Geometry: see drawing. Coordinates: mm, zero at the bounding-box minimum. Round coordinates to 2 decimals unless told otherwise and drop trailing zeros. Order: outer loops, then holes, each group sorted by start corner. A loop starts at its lowest first (then second) coordinate and runs counter-clockwise, first axis right, second up. Notation, with made-up numbers: (18.25, -8.5) -> (72.25, -8.5) arc R13 cw to (72.25, 16.5) -> close; hole circle Ø6 at (40.25, 57.5). An arc over 180 degrees is marked (long way). Answer as CSV lines item,"result". Start each with the question number.
(1) Section query B-B (y = 10.16). Output: boundary loops of the cut face in (x, z) (3 decimals).
(2) Section query A-A (x = 12.7). Output: boundary loops of the cut face in (y, z) (3 decimals).
(3) Section query C-C (z = 2.45). Output: boundary loops of the cut face in (x, y), plus the area to 3 significant figures.
(4) Line query: line 1 along Y through (x, z) = (38.1, 0.9); line 2 along X through (y, z) = (10.16, 0.7); line 3 along Y through (x, z) = (39.5, 2.4). Output: solid intervals per line, ascending. Write a range as from..to.
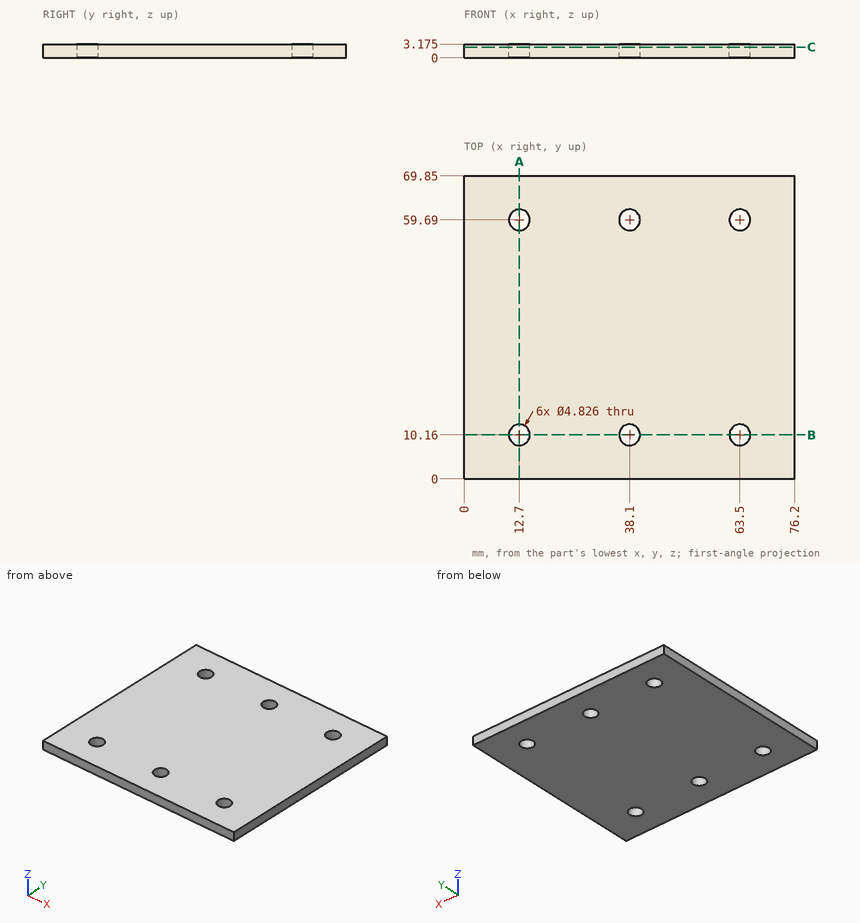
Answer block:
1,outline,"(0, 0) -> (10.287, 0) -> (10.287, 3.175) -> (0, 3.175) -> close; (15.113, 0) -> (35.687, 0) -> (35.687, 3.175) -> (15.113, 3.175) -> close; (40.513, 0) -> (61.087, 0) -> (61.087, 3.175) -> (40.513, 3.175) -> close; (65.913, 0) -> (76.2, 0) -> (76.2, 3.175) -> (65.913, 3.175) -> close"
2,outline,"(0, 0) -> (7.747, 0) -> (7.747, 3.175) -> (0, 3.175) -> close; (12.573, 0) -> (57.277, 0) -> (57.277, 3.175) -> (12.573, 3.175) -> close; (62.103, 0) -> (69.85, 0) -> (69.85, 3.175) -> (62.103, 3.175) -> close"
3,outline,"(0, 0) -> (76.2, 0) -> (76.2, 69.85) -> (0, 69.85) -> close; hole circle Ø4.83 at (12.7, 10.16); hole circle Ø4.83 at (12.7, 59.69); hole circle Ø4.83 at (38.1, 10.16); hole circle Ø4.83 at (38.1, 59.69); hole circle Ø4.83 at (63.5, 10.16); hole circle Ø4.83 at (63.5, 59.69)"
3,area,"5,210 mm2"
4,line 1,"0..7.75, 12.57..57.28, 62.1..69.85"
4,line 2,"0..10.29, 15.11..35.69, 40.51..61.09, 65.91..76.2"
4,line 3,"0..8.19, 12.13..57.72, 61.66..69.85"
